from build123d import *

# Parameters (mm, degrees)
SKETCH1_R           = 1.7
SKETCH1_R_2         = 1.65
BOSS_EXTRUDE1_DEPTH = 3
CHAMFER2_SIZE       = 0.5
SKETCH2_W           = 9
SKETCH2_H           = 12
BOSS_EXTRUDE2_DEPTH = 17
SKETCH3_R           = 2.5
CUT_EXTRUDE1_DEPTH  = 2
SKETCH4_R           = 2.5
SKETCH4_R_2         = 1.7
BOSS_EXTRUDE3_DEPTH = 3


with BuildPart() as part:
    # Sketch1 → Boss-Extrude1 (new body)
    with BuildSketch(Plane.XY):
        with BuildLine():
            Line((20, 20), (20, -20))
            Line((20, -20), (-15.784232335, -20))
            Line((-15.784232335, -20), (-27.5, -26.764101615))
            ThreePointArc((-27.5, -26.764101615), (-30.022104769, -27.265779445), (-32.328427125, -26.128427125))
            Line((-32.328427125, -26.128427125), (-67.328427125, 8.871572875))
            ThreePointArc((-67.328427125, 8.871572875), (-68.264653884, 13.051806618), (-64.883087414, 15.681613245))
            Line((-64.883087414, 15.681613245), (-20, 20))
            Line((-20, 20), (-4, 20))
            Line((-4, 20), (-4, 35))
            Line((-4, 35), (20, 35))
            Line((20, 35), (20, 20))
        make_face()
        with Locations((-17, 17)):
            Circle(SKETCH1_R, mode=Mode.SUBTRACT)
        with Locations((17, 17)):
            Circle(SKETCH1_R, mode=Mode.SUBTRACT)
        with Locations((17, -17)):
            Circle(SKETCH1_R, mode=Mode.SUBTRACT)
        with Locations((-17, -17)):
            Circle(SKETCH1_R, mode=Mode.SUBTRACT)
        with Locations((0.15, 31)):
            Circle(SKETCH1_R, mode=Mode.SUBTRACT)
        with Locations((15.75, 31)):
            Circle(SKETCH1_R, mode=Mode.SUBTRACT)
        with Locations((-64.5, 11.7)):
            Circle(SKETCH1_R_2, mode=Mode.SUBTRACT)
        with Locations((-29.5, -23.3)):
            Circle(SKETCH1_R_2, mode=Mode.SUBTRACT)
    extrude(amount=BOSS_EXTRUDE1_DEPTH)

    # Chamfer2
    chamfer2_edges = [part.edges().sort_by_distance(p)[0] for p in [
        (-66.15, 11.7, 3),
    ]]
    chamfer(chamfer2_edges, length=CHAMFER2_SIZE)

    # Sketch2 → Boss-Extrude2 (add)
    with BuildSketch(Plane.XY.offset(3)):
        with Locations((7.95, 29)):
            Rectangle(SKETCH2_W, SKETCH2_H)
    extrude(amount=BOSS_EXTRUDE2_DEPTH)

    # Sketch3 → Cut-Extrude1 (cut)
    with BuildSketch(Plane.XY.offset(20)):
        with Locations((7.95, 29)):
            Circle(SKETCH3_R)
    extrude(amount=-CUT_EXTRUDE1_DEPTH, mode=Mode.SUBTRACT)

    # Sketch4 → Boss-Extrude3 (add)
    # profile 1 of 4: a face of its own
    with BuildSketch(Plane.XY.offset(3)):
        with Locations((-17, 17)):
            Circle(SKETCH4_R)
        with Locations((-17, 17)):
            Circle(SKETCH4_R_2, mode=Mode.SUBTRACT)
    # profile 2 of 4: a face of its own
    with BuildSketch(Plane.XY.offset(3)):
        with Locations((17, 17)):
            Circle(SKETCH4_R)
        with Locations((17, 17)):
            Circle(SKETCH4_R_2, mode=Mode.SUBTRACT)
    # profile 3 of 4: a face of its own
    with BuildSketch(Plane.XY.offset(3)):
        with Locations((-17, -17)):
            Circle(SKETCH4_R)
        with Locations((-17, -17)):
            Circle(SKETCH4_R_2, mode=Mode.SUBTRACT)
    # profile 4 of 4: a face of its own
    with BuildSketch(Plane.XY.offset(3)):
        with Locations((17, -17)):
            Circle(SKETCH4_R)
        with Locations((17, -17)):
            Circle(SKETCH4_R_2, mode=Mode.SUBTRACT)
    extrude(amount=BOSS_EXTRUDE3_DEPTH)


solid = part.part
Read the model definition and answer for the solid it produces. Units are mm, in the model's axes. A direction names the side the tool comes from. Give positions to 0.01 mm unless a question says otherwise; leave off trailing zeros. Loops run counter-clockwise (first coordinate to the right, second up) from the corner with the lowest first, then second, coordinate; pieces in that order, holes last. Notation, with made-up numbers: (29, 42) -> (63, 42) arc R23 ccw to (63, 59) -> close; hole circle Ø5 at (-23, 18.25). An arc over 180 degrees is marked (long way). Use a Markdown table: item, result.
Q1. A tool of negligible diameter and unlimited length cuts with its end or side. For faces 5 (the face through (12.45, 29, 11)), 6 (the face through (2, -20, 1)), 7 (the face through (14.5, -16.9, 4.5)), from which of +Z, -Z, +X, -X, +Y, -Y can it reach the whole face along a straight path? Write none if from no direction.
Solved:
| item | result |
|---|---|
| face 5 | +Z, +X, +Y, -Y |
| face 6 | +Z, -Z, +X, -Y |
| face 7 | +Z |
Q2. Section A-A, the plane z = 4 is taken. Count the separate pieces of the cut face and the enclosed holes in it, then the cut area to 3 significant figures.
Solved:
| item | result |
|---|---|
| separate pieces | 5 |
| enclosed holes | 4 |
| area | 150 mm^2 |
Q3. Determine the mould class of faces 1 (the face through (3.45, 29, 11)), 2 (the face through (8, 29, 18)), 3 (the face through (-16, 15, 6)), 4 (the face through (-19.5, 17.1, 4.5)) for opening direction X: pulls with the +X half, pulls with the -X half, needs draft (parallel to the pull), parting line crosses it, or undercut.
Solved:
| item | result |
|---|---|
| face 1 | pulls with the -X half |
| face 2 | undercut |
| face 3 | needs draft |
| face 4 | undercut |
Q4. Section D-D, the plane y = -17 is taken. Determine the outline of the cut face in (x, z), then the cut area to 3 significant figures.
Solved:
| item | result |
|---|---|
| outline | (-41.46, 0) -> (-18.7, 0) -> (-18.7, 6) -> (-19.5, 6) -> (-19.5, 3) -> (-41.46, 3) -> close; (-15.3, 0) -> (15.3, 0) -> (15.3, 6) -> (14.5, 6) -> (14.5, 3) -> (-14.5, 3) -> (-14.5, 6) -> (-15.3, 6) -> close; (18.7, 0) -> (20, 0) -> (20, 3) -> (19.5, 3) -> (19.5, 6) -> (18.7, 6) -> close |
| area | 174 mm^2 |
Q5. Find the intervals of material crossed by line 1 along Y through (x, z) = (17, 4.4); line 2 along X through (y, z) = (18, 5.5); line 3 along Z through (x, y) = (-44.5, 1.5), in increasing order.
Solved:
| item | result |
|---|---|
| line 1 | y = -19.5 to -18.7, -15.3 to -14.5, 14.5 to 15.3, 18.7 to 19.5 |
| line 2 | x = -19.29 to -18.37, -15.63 to -14.71, 14.71 to 15.63, 18.37 to 19.29 |
| line 3 | z = 0 to 3 |
Q6. Section B-B, the plane x = 0.15 is taken. Determine the outline of the cut face in (y, z), then the cut area to 3 significant figures.
Solved:
| item | result |
|---|---|
| outline | (-20, 0) -> (29.3, 0) -> (29.3, 3) -> (-20, 3) -> close; (32.7, 0) -> (35, 0) -> (35, 3) -> (32.7, 3) -> close |
| area | 155 mm^2 |
Q7. Each of these flat-tipped pins is pushed along its axis until it touches: pin 1 (3 mm diameter, centred on x = 6.5, y = 13, fed in from +Z); pin 2 (3.5 mm diameter, centred on y = 30, z = 8.5, fed in from +X); pin 3 (2.5 mm diameter, centred on x = 0.15, y = 31, fed in from -Z); pin 4 (2.5 mm diameter, centred on x = -3, z = 2, fed in from -Y). Where does it stop, or does it pass through?
Solved:
| item | result |
|---|---|
| pin 1 | stops at z = 3 |
| pin 2 | stops at x = 12.45 |
| pin 3 | passes through |
| pin 4 | stops at y = -20 |
Q8. Section C-C, the plane y = 11.7 is taken. Determine the outline of the cut face in (x, z).
Solved:
| item | result |
|---|---|
| outline | (-68.5, 0) -> (-66.15, 0) -> (-66.15, 2.5) -> (-66.65, 3) -> (-68.5, 3) -> close; (-62.85, 0) -> (20, 0) -> (20, 3) -> (-62.35, 3) -> (-62.85, 2.5) -> close |
